Work out the finished part from the listing and answer in its coordinate system (mm). A direction names the side the tool comes from. Coordinates: 2 decimals unless noted, no trailing zeros. Order: outer loops, then holes, each group sorted by start corner. A loop starts at its lowest first (then second) coordinate and runs counter-clockwise, first axis right, second up. Notation, with made-up numbers: M -25,29 L 28,29 A21 cw 28,67 Z; hole C 21.25,-33 d8. An arc over 180 degrees is marked long. Use a Markdown table: item, result.
from build123d import *

# Parameters (mm, degrees)
SKETCH1_R           = 1.35
BOSS_EXTRUDE1_DEPTH = 46.736
SKETCH2_W           = 76.454
SKETCH2_H           = 38.354
CUT_EXTRUDE1_DEPTH  = 137.16
FILLET1_R           = 2.54
SKETCH3_R           = 3.05
CUT_EXTRUDE2_DEPTH  = 66.294


with BuildPart() as part:
    # Sketch1 → Boss-Extrude1 (new body)
    with BuildSketch(Plane.XY):
        Polygon((-53.90661, 47), (-53.90661, -7), (20, -7), (20, -48.25), (106.614, -48.25), (106.614, 53.35), (20, 53.35), (20, 47), align=None)
        Circle(SKETCH1_R, mode=Mode.SUBTRACT)
        with Locations((-27, 0)):
            Circle(SKETCH1_R, mode=Mode.SUBTRACT)
        with Locations((-45.90661, 0.5)):
            Circle(SKETCH1_R, mode=Mode.SUBTRACT)
        with Locations((-45.90661, 27.5)):
            Circle(SKETCH1_R, mode=Mode.SUBTRACT)
        with Locations((-27, 28)):
            Circle(SKETCH1_R, mode=Mode.SUBTRACT)
        with Locations((0, 28)):
            Circle(SKETCH1_R, mode=Mode.SUBTRACT)
    extrude(amount=BOSS_EXTRUDE1_DEPTH)

    # Sketch2 → Cut-Extrude1 (cut)
    with BuildSketch(Plane(origin=(0, 53.35, 0), x_dir=(1, 0, 0), z_dir=(0, 1, 0))):
        Polygon((-53.90661, -7.62), (4.51339, -7.62), (9.59339, -12.7), (9.59339, -34.036), (4.51339, -39.116), (-53.90661, -39.116), align=None)
        with Locations((63.307, -23.368)):
            Rectangle(SKETCH2_W, SKETCH2_H)
    extrude(amount=-CUT_EXTRUDE1_DEPTH, mode=Mode.SUBTRACT)

    # Fillet1
    fillet1_edges = [part.edges().sort_by_distance(p)[0] for p in [
        (20, 50.175, 0),
        (-53.90661, -7, 42.926),
        (-53.90661, 47, 42.926),
        (20, -27.625, 46.736),
        (106.614, 2.55, 46.736),
        (-53.90661, -7, 3.81),
        (-53.90661, 47, 3.81),
        (4.51339, 20, 7.62),
        (9.59339, 20, 12.7),
        (9.59339, 20, 34.036),
        (4.51339, 20, 39.116),
        (106.614, 2.55, 0),
        (20, 50.175, 46.736),
        (20, -27.625, 0),
    ]]
    fillet(fillet1_edges, radius=FILLET1_R)

    # Sketch3 → Cut-Extrude2 (cut)
    with BuildSketch(Plane.XY.offset(46.736)):
        with Locations((63.307, 27.95)):
            Circle(SKETCH3_R)
        with Locations((63.307, -22.85)):
            Circle(SKETCH3_R)
    extrude(amount=-CUT_EXTRUDE2_DEPTH, mode=Mode.SUBTRACT)


solid = part.part
1. Find the intervals of material crossed by probe 1 along Y at (x, z) = (-27, 42.5); probe 2 along X at (y, z) = (-27, 19.5); probe 3 along Z at (x, y) = (71, 34) (3 decimals), in increasing order.
Answers below:
| item | result |
|---|---|
| probe 1 | -7 to -1.35, 1.35 to 26.65, 29.35 to 47 |
| probe 2 | 20 to 25.08, 101.53 to 106.61 |
| probe 3 | 0 to 4.191, 42.545 to 46.736 |
2. Section A-A on x = -6 is taken. Determine the outline of the cut face in (y, z), then the cut area to 3 significant figures.
Answers below:
| item | result |
|---|---|
| outline | M -7,0 L 47,0 L 47,7.62 L -7,7.62 Z; M -7,39.12 L 47,39.12 L 47,46.74 L -7,46.74 Z |
| area | 823 mm² |
3. Section C-C on y = -22.85 is taken. Determine the outline of the cut face in (x, z) (3 decimals), then the cut area to 3 significant figures.
Answers below:
| item | result |
|---|---|
| outline | M 20,2.54 A2.54 ccw 22.54,0 L 60.257,0 L 60.257,4.191 L 25.08,4.191 L 25.08,42.545 L 60.257,42.545 L 60.257,46.736 L 22.54,46.736 A2.54 ccw 20,44.196 Z; M 66.357,0 L 104.074,0 A2.54 ccw 106.614,2.54 L 106.614,44.196 A2.54 ccw 104.074,46.736 L 66.357,46.736 L 66.357,42.545 L 101.534,42.545 L 101.534,4.191 L 66.357,4.191 Z |
| area | 1,060 mm² |
4. For faces 1 (the face through (9.593, 20, 23)), 2 (the face through (20, -27, 23)), 3 (the face through (25.08, 3, 24)), determine the directions among +Z, -Z, +X, -X, +Y, -Y from which every point of the face is accessible in a straight line to the end or side of a thin tool.
Answers below:
| item | result |
|---|---|
| face 1 | -X, +Y, -Y |
| face 2 | +Z, -Z, -X, -Y |
| face 3 | +Y, -Y |
5. Section D-D on x = 93 is taken. Determine the outline of the cut face in (y, z) (3 decimals).
Answers below:
| item | result |
|---|---|
| outline | M -48.25,0 L 53.35,0 L 53.35,4.191 L -48.25,4.191 Z; M -48.25,42.545 L 53.35,42.545 L 53.35,46.736 L -48.25,46.736 Z |
6. Flat-ended cylindrical pins translate along their axes: P1, Ø1.6, axis at x = -45.91, y = 27.5, coming from the +Z side; P2, Ø7, axis at y = 51, z = 28.5, coming from the -X side. Find the tip coordinate at first contact, or state that the pin passes through.
Answers below:
| item | result |
|---|---|
| P1 | through |
| P2 | x = 20 |
7. Section B-B on z = 26.5 is taken. Determine the outline of the cut face in (x, y), then the cut area to 3 significant figures.
Answers below:
| item | result |
|---|---|
| outline | M 9.59,-7 L 20,-7 L 20,-48.25 L 25.08,-48.25 L 25.08,53.35 L 20,53.35 L 20,47 L 9.59,47 Z; M 101.53,-48.25 L 106.61,-48.25 L 106.61,53.35 L 101.53,53.35 Z |
| area | 1,590 mm² |
8. For a pull along X with two mould halves and no side action, classify faces 4 (the face through (61.06, 30.01, 2.12)), 5 (the face through (60.89, -24.71, 2.12)), 6 (the face through (7.08, 20.38, 36.55)), 7 (the face through (42, 3, 46.736)) as +X half, -X half, draft (parallel to the pull), parting line (faces both ways), or undercut.
Answers below:
| item | result |
|---|---|
| face 4 | undercut |
| face 5 | undercut |
| face 6 | -X half |
| face 7 | draft |
